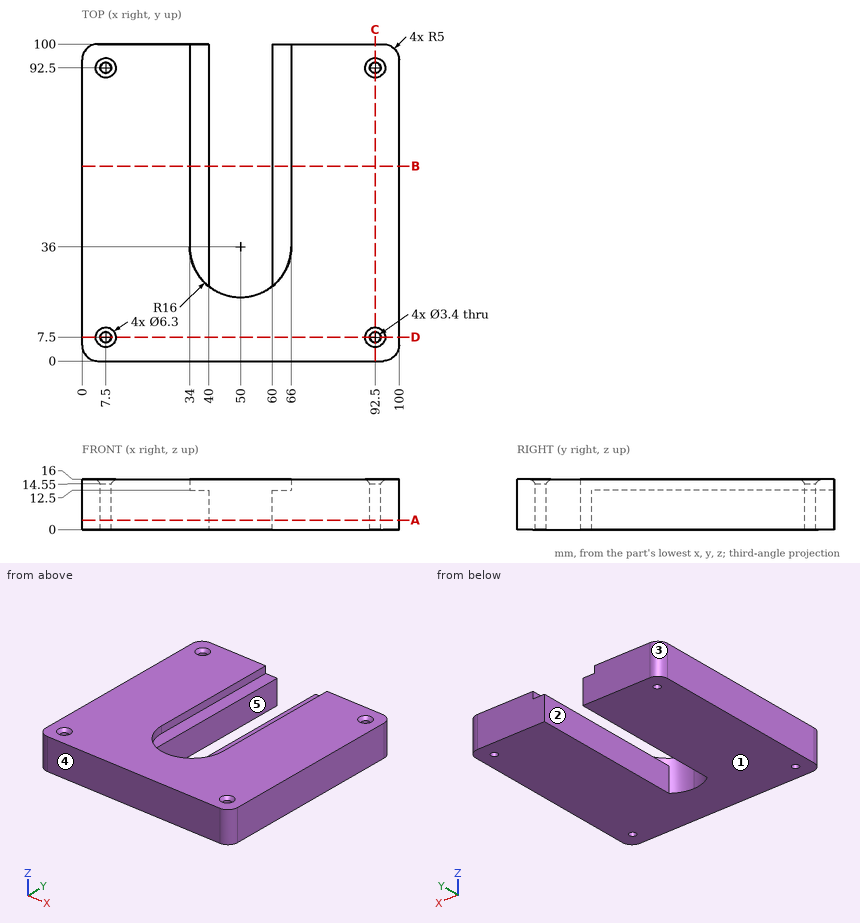
Here's the drawing with two shaded views (mm, measured from the low corner). I have some questions. A direction names the side the tool comes from. Coordinates: 2 decimals unless noted, no trailing zeros. Order: outer loops, then holes, each group sorted by start corner. A loop starts at its lowest first (then second) coordinate and runs counter-clockwise, first axis right, second up.
Item 1: For the marked faces 4 and 5, which set-ups out of +Z, -Z, +X, -X, +Y, -Y let a thin tool reach every point of the face, with its end or its side?
Result sheet:
face 4: +Z, -Z, +X, -X, -Y
face 5: +Z, -Z, +Y
Item 2: If we section it at B-B on y = 61.5: List the corners of the cut face in (x, z) for me.
Result sheet:
outline: (0, 0) - (40, 0) - (40, 12.5) - (34, 12.5) - (34, 16) - (0, 16) - close; (60, 0) - (100, 0) - (100, 16) - (66, 16) - (66, 12.5) - (60, 12.5) - close
Item 3: For P1, Ø4.5, axis at x = 92.5, y = 92.5, coming from the +Z side; P2, Ø3, axis at x = 63, y = 56.5, coming from the +Z side; P3, Ø2, axis at x = 7.5, y = 7.5, coming from the -Z side, each with a flat end and sliding along its axis, tell me the tip position at first contact or that it passes through.
Result sheet:
P1: stops at z = 15.1
P2: stops at z = 12.5
P3: passes through
Item 4: If we section it at C-C on x = 92.5: List the corners of the cut face in (y, z) for me, plus the area to 3 significant figures.
Result sheet:
outline: (0, 0) - (5.8, 0) - (5.8, 14.55) - (4.35, 16) - (0, 16) - close; (9.2, 0) - (90.8, 0) - (90.8, 14.55) - (89.35, 16) - (10.65, 16) - (9.2, 14.55) - close; (94.2, 0) - (100, 0) - (100, 16) - (95.65, 16) - (94.2, 14.55) - close
area: 1,490 mm2
Item 5: If we mould it in two halves opening along X, with no side actions, what happens to the marked faces 1, 2 and 3? For each: +X half, -X half, draft (parallel to the pull), parting line (faces both ways), or undercut.
Result sheet:
face 1: draft
face 2: undercut
face 3: -X half
Item 6: I need wall thicknesses on line 1 (X direction, y = 92.5, z = 11); line 2 (Y direction, x = 7.5, z = 4.75). Which ranges of each line are inside material? Lowest first, please.
Result sheet:
line 1: x = 0 to 5.8, 9.2 to 40, 60 to 90.8, 94.2 to 100
line 2: y = 0 to 5.8, 9.2 to 90.8, 94.2 to 100
Item 7: If we section it at A-A on z = 3: List the corners of the cut face in (x, y) for me.
Result sheet:
outline: (0, 5) arc R5 ccw to (5, 0) - (95, 0) arc R5 ccw to (100, 5) - (100, 95) arc R5 ccw to (95, 100) - (60, 100) - (60, 23.51) arc R16 cw to (40, 23.51) - (40, 100) - (5, 100) arc R5 ccw to (0, 95) - close; hole circle Ø3.4 at (7.5, 7.5); hole circle Ø3.4 at (7.5, 92.5); hole circle Ø3.4 at (92.5, 7.5); hole circle Ø3.4 at (92.5, 92.5)
